Design review of the part shown in the three views and the two pictorial views. Dimensions are in mm from the part's minimum x, y and z. Coordinates: 2 decimals unless noted, no trailing zeros. Write each loop counter-clockwise with the first axis right and the second up, starting at its lowest first coordinate (ties: lowest second). Pieces come first, ordered by that corner, then holes. Notation, with made-up numbers: (49.5, 63) - (60.5, 63) arc R32 ccw to (60.5, 101) - close; hole circle Ø6 at (15, 65.5). An arc over 180 degrees is marked (long way). Return JSON: item names as keys, results as strings. Group by question number.
(1) To check wall thickness, follow L1, parallel to Y at x = 4, z = 0.8; L2, parallel to X at y = 6.25, z = 1.4; L3, parallel to Y at x = 14.5, z = 0.2. State the ranges of each line that lie inside material, in increasing order. Write a range as from..to.
(2) We need section D-D on x = 14. State the section outline as (y, z) points, then the cut area to 3 significant figures.
(3) We need section A-A on z = 0.25. State the section outline as (x, y) points, then the cut area to 3 significant figures.
(4) We need section B-B on y = 13.25. State the section outline as (x, z) points.
(5) For pin 1 Ø2.5 at (x, y) = (8, 7.5) entering from +Z; pin 2 Ø1.2 at (x, y) = (4, 7.5) entering from +Z, all flat-tipped, find the tip position at first contact; note any pin that passes through.
(6) We need section C-C on x = 1.75. State the section outline as (y, z) points.
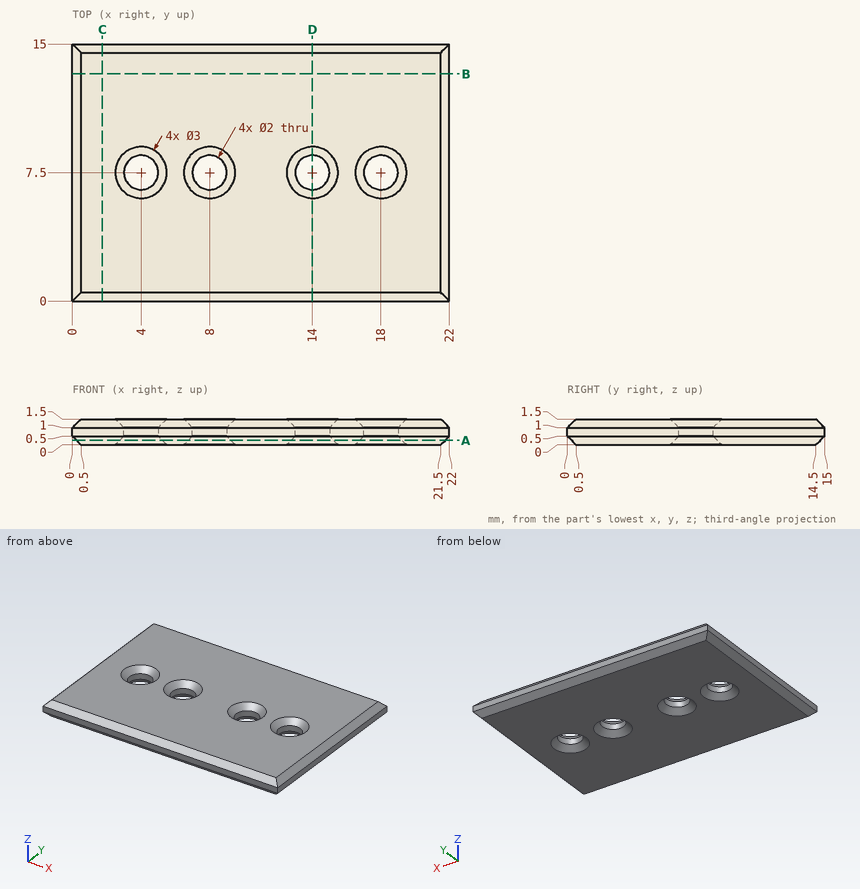
Ans:
{
 "1": {"L1": "0..6.5, 8.5..15", "L2": "0.4..3.37, 4.63..7.37, 8.63..13.37, 14.63..17.37, 18.63..21.6", "L3": "0.3..6.3, 8.7..14.7"},
 "2": {"outline": "(0, 0.5) - (0.5, 0) - (6, 0) - (6.5, 0.5) - (6.5, 1) - (6, 1.5) - (0.5, 1.5) - (0, 1) - close; (8.5, 0.5) - (9, 0) - (14.5, 0) - (15, 0.5) - (15, 1) - (14.5, 1.5) - (9, 1.5) - (8.5, 1) - close", "area": "18.5 mm²"},
 "3": {"outline": "(0.25, 0.25) - (21.75, 0.25) - (21.75, 14.75) - (0.25, 14.75) - close; hole circle Ø2.5 at (4, 7.5); hole circle Ø2.5 at (8, 7.5); hole circle Ø2.5 at (14, 7.5); hole circle Ø2.5 at (18, 7.5)", "area": "292 mm²"},
 "4": {"outline": "(0, 0.5) - (0.5, 0) - (21.5, 0) - (22, 0.5) - (22, 1) - (21.5, 1.5) - (0.5, 1.5) - (0, 1) - close"},
 "5": {"pin 1": "z = 1.25", "pin 2": "through"},
 "6": {"outline": "(0, 0.5) - (0.5, 0) - (14.5, 0) - (15, 0.5) - (15, 1) - (14.5, 1.5) - (0.5, 1.5) - (0, 1) - close"}
}
